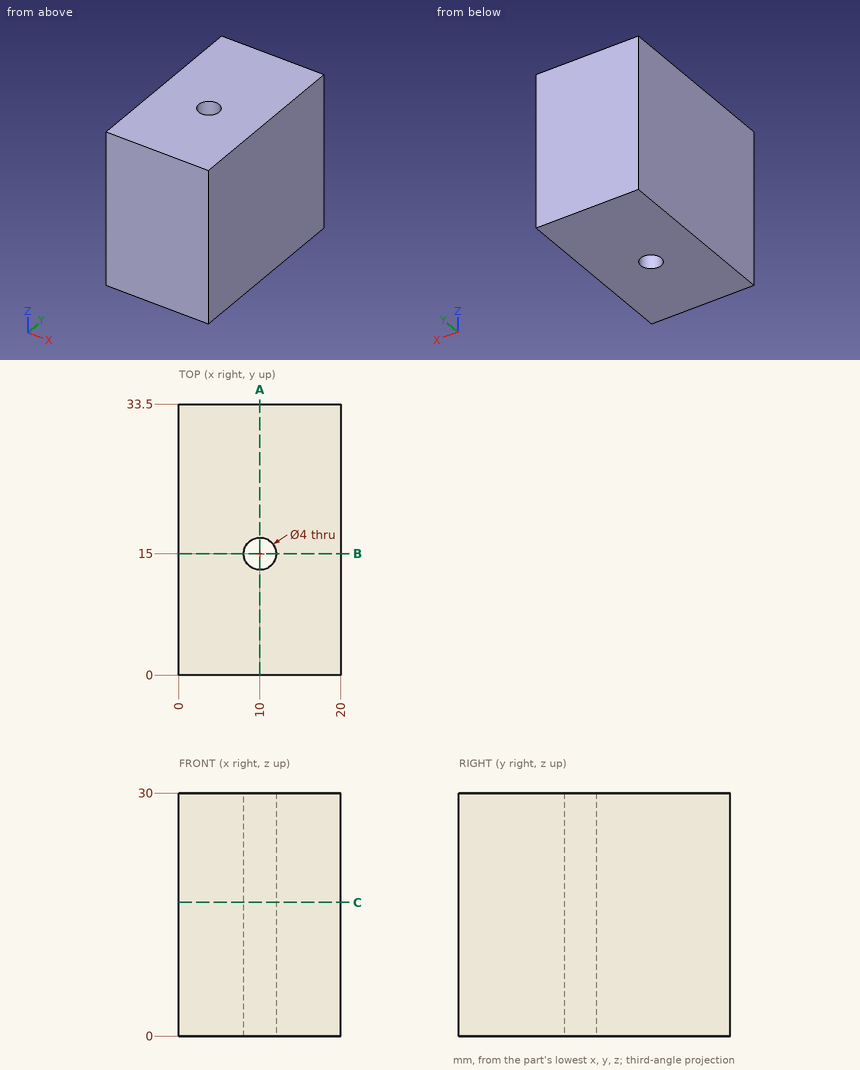
The figure shows three views and two pictorial views of one solid part (mm, origin at its lowest corner). Answer the questions. Round coordinates to 2 decimals unless told otherwise and drop trailing zeros. Order: outer loops, then holes, each group sorted by start corner. A loop starts at its lowest first (then second) coordinate and runs counter-clockwise, first axis right, second up. Notation, with made-up numbers: M -19,-24.75 L 34,-24.75 A18 ccw 34,-15.75 Z; hole C 88.25,6 d2. An arc over 180 degrees is marked long. Answer in a Markdown table with one row per item. Add a question column.
1) The part is cut by section C-C on z = 16.5. Determine the outline of the cut face in (x, y), plus the area to 3 significant figures.
2) Consider line 1 along Y through (x, z) = (10, 8.25); line 2 along X through (y, z) = (16.5, 28.75); line 3 along X through (y, z) = (16, 28.75). Determine where each line is inside the solid, lowest interval first. Write a range as from..to.
3) The part is cut by section B-B on y = 15. Determine the outline of the cut face in (x, z).
4) The part is cut by section A-A on x = 10. Determine the outline of the cut face in (y, z).
Findings below:
| question | item | result |
|---|---|---|
| 1 | outline | M 0,0 L 20,0 L 20,33.5 L 0,33.5 Z; hole C 10,15 d4 |
| 1 | area | 657 mm² |
| 2 | line 1 | y = 0..13, 17..33.5 |
| 2 | line 2 | x = 0..8.68, 11.32..20 |
| 2 | line 3 | x = 0..8.27, 11.73..20 |
| 3 | outline | M 0,0 L 8,0 L 8,30 L 0,30 Z; M 12,0 L 20,0 L 20,30 L 12,30 Z |
| 4 | outline | M 0,0 L 13,0 L 13,30 L 0,30 Z; M 17,0 L 33.5,0 L 33.5,30 L 17,30 Z |
